from build123d import *

# Parameters (mm, degrees)
SKETCH1_W           = 63
SKETCH1_H           = 65
BOSS_EXTRUDE1_DEPTH = 35
SKETCH4_W           = 13.85
SKETCH4_H           = 28
CUT_EXTRUDE1_DEPTH  = 81.26362829
SKETCH6_R           = 2.05
CUT_EXTRUDE2_DEPTH  = 35
SKETCH7_W           = 35.3
SKETCH7_H           = 20
CUT_EXTRUDE3_DEPTH  = 58.214508823
SKETCH5_W           = 43.787246082
SKETCH5_H           = 26.488580963
CUT_EXTRUDE4_DEPTH  = 81.26362829
FILLET1_R           = 3
FILLET2_R           = 5


with BuildPart() as part:
    # Sketch1 → Boss-Extrude1 (new body)
    with BuildSketch(Plane.XY):
        Rectangle(SKETCH1_W, SKETCH1_H)
    extrude(amount=BOSS_EXTRUDE1_DEPTH)

    # Cut-Loft1: read off the stored shape, not the designer's step
    # Cut-Loft1: loft between two sections, ruled curve by curve
    cut_loft1_from = [
        Edge.make_bspline([(-16.5, -32.5, -15.95), (-16.5, -32.5, -14.245344374), (-16.5, -32.5, -10.830534175), (-16.5, -32.5, -5.7), (-16.5, -32.5, -0.569465825), (-16.5, -32.5, 2.845344374), (-16.5, -32.5, 5.208176172), (-16.24079277, -32.5, 6.487165764), (-15.189486136, -32.5, 8.102764154), (-13.584460954, -32.5, 9.238586175), (-12.225257815, -32.5, 9.55), (-9.654092683, -32.5, 9.55), (-5.862169747, -32.5, 9.55), (0, -32.5, 9.55), (5.862169747, -32.5, 9.55), (9.654092683, -32.5, 9.55), (12.225257815, -32.5, 9.55), (13.584460954, -32.5, 9.238586175), (15.189486136, -32.5, 8.102764154), (16.24079277, -32.5, 6.487165764), (16.5, -32.5, 5.208176172), (16.5, -32.5, 4.55)], [0, 0, 0, 0, 0.090746911, 0.181493823, 0.272240734, 0.362987645, 0.362987645, 0.398025487, 0.43306333, 0.468101172, 0.503139015, 0.503139015, 0.592316419, 0.681493823, 0.770671227, 0.859848631, 0.859848631, 0.894886473, 0.929924315, 0.964962158, 1, 1, 1, 1], 3),
        Edge.make_line((16.5, -32.5, 0), (16.5, -32.5, 4.55)),
        Edge.make_line((16.5, -32.5, 0), (-16.5, -32.5, -15.95)),
    ]
    cut_loft1_to = [
        Edge.make_bspline([(-13.65, 32.5, -15.8), (-13.65, 32.5, -14.113380525), (-13.65, 32.5, -10.745084998), (-13.65, 32.5, -5.7), (-13.65, 32.5, -0.654915002), (-13.65, 32.5, 2.713380525), (-13.65, 32.5, 5.051212323), (-13.38927185, 32.5, 6.394463384), (-12.20097724, 32.5, 8.116532102), (-10.480556624, 32.5, 9.187425671), (-9.241272853, 32.5, 9.4), (-7.145107721, 32.5, 9.4), (-4.236047985, 32.5, 9.4), (0, 32.5, 9.4), (4.236047985, 32.5, 9.4), (7.145107721, 32.5, 9.4), (9.241272853, 32.5, 9.4), (10.480556624, 32.5, 9.187425671), (12.20097724, 32.5, 8.116532102), (13.38927185, 32.5, 6.394463384), (13.65, 32.5, 5.051212323), (13.65, 32.5, 4.4)], [0, 0, 0, 0, 0.090746911, 0.181493823, 0.272240734, 0.362987645, 0.362987645, 0.398025487, 0.43306333, 0.468101172, 0.503139015, 0.503139015, 0.592316419, 0.681493823, 0.770671227, 0.859848631, 0.859848631, 0.894886473, 0.929924315, 0.964962158, 1, 1, 1, 1], 3),
        Edge.make_line((13.65, 32.5, 0), (13.65, 32.5, 4.4)),
        Edge.make_line((13.65, 32.5, 0), (-13.65, 32.5, -15.8)),
    ]
    cut_loft1 = Solid(Shell([*[Face.make_surface_from_curves(cut_loft1_from[k], cut_loft1_to[k]) for k in range(3)], Face(Wire(cut_loft1_from)), Face(Wire(cut_loft1_to))]))
    add(cut_loft1, mode=Mode.SUBTRACT)

    # Sketch4 → Cut-Extrude1 (cut, through all)
    with BuildSketch(Plane(origin=(0, 32.5, 0), x_dir=(1, 0, 0), z_dir=(0, 1, 0))):
        with Locations((24.575, -21)):
            Rectangle(SKETCH4_W, SKETCH4_H)
        with Locations((-24.575, -21)):
            Rectangle(SKETCH4_W, SKETCH4_H)
    extrude(amount=-CUT_EXTRUDE1_DEPTH, mode=Mode.SUBTRACT)

    # Sketch6 → Cut-Extrude2 (cut)
    with BuildSketch(Plane(origin=(0, 0, 0), x_dir=(-1, 0, 0), z_dir=(0, 0, -1))):
        with Locations((-26.5, -18.5)):
            Circle(SKETCH6_R)
        with Locations((-26.5, 1.5)):
            Circle(SKETCH6_R)
        with Locations((-26.5, 21.5)):
            Circle(SKETCH6_R)
        with Locations((26.5, -18.5)):
            Circle(SKETCH6_R)
        with Locations((26.5, 1.5)):
            Circle(SKETCH6_R)
        with Locations((26.5, 21.5)):
            Circle(SKETCH6_R)
    extrude(amount=-CUT_EXTRUDE2_DEPTH, mode=Mode.SUBTRACT)

    # Sketch7 → Cut-Extrude3 (cut, through all)
    with BuildSketch(Plane.XY.offset(35)):
        with Locations((0, -22.5)):
            Rectangle(SKETCH7_W, SKETCH7_H)
    extrude(amount=-CUT_EXTRUDE3_DEPTH, mode=Mode.SUBTRACT)

    # Sketch5 → Cut-Extrude4 (cut, through all)
    with BuildSketch(Plane(origin=(0, 32.5, 0), x_dir=(1, 0, 0), z_dir=(0, 1, 0))):
        with Locations((-0.216233314, -27.644290482)):
            Rectangle(SKETCH5_W, SKETCH5_H)
    extrude(amount=-CUT_EXTRUDE4_DEPTH, mode=Mode.SUBTRACT)

    # Fillet1
    fillet1_edges = [part.edges().sort_by_distance(p)[0] for p in [
        (17.65, 10, 7),
        (-17.65, 10, 7),
    ]]
    fillet(fillet1_edges, radius=FILLET1_R)

    # Fillet2
    fillet2_edges = [part.edges().sort_by_distance(p)[0] for p in [
        (-17.65, 10, 14.4),
        (17.65, 10, 14.4),
    ]]
    fillet(fillet2_edges, radius=FILLET2_R)


solid = part.part
Work out the finished part from the listing and answer in its coordinate system (mm). A direction names the side the tool comes from. Give positions to 0.01 mm unless a question says otherwise; leave off trailing zeros. Order: outer loops, then holes, each group sorted by start corner. A loop starts at its lowest first (then second) coordinate and runs counter-clockwise, first axis right, second up. Notation, with made-up numbers: (-36, 7.5) -> (4, 7.5) arc R33 ccw to (4, 46.5) -> close; hole circle Ø2 at (10, 2.25). An arc over 180 degrees is marked (long way). One line per item, written item: value.
Item 1: Determine the mould class of faces 3 (the cylindrical face through (28, -17.1, 3.5)), 4 (the flat face through (0, 10, 14.4)), 5 (the flat face through (-25, -32.5, 3)), 6 (the cylindrical face through (-24.45, 1.59, 3.45)) for opening direction Y: released by +Y, released by -Y, zero draft, split by the parting line, or undercut.
Answer sheet:
face 3: undercut
face 4: zero draft
face 5: released by -Y
face 6: undercut
Item 2: Straight lines are drawn through the part: probe 1 along Y at (x, z) = (-26.5, 3); probe 2 along X at (y, z) = (-25, 4); probe 3 along Y at (x, z) = (16, 2.25). For each, find the intervals that lie inside material, in ascending order.
Answer sheet:
probe 1: -32.5 to -20.55, -16.45 to -0.55, 3.55 to 19.45, 23.55 to 32.5
probe 2: -31.5 to -17.65, 17.65 to 31.5
probe 3: -12.5 to 32.5
Item 3: Find section A-A, the plane y = -18.5. Give the vertices of the cut face in (x, z), plus the area to 4 significant figures.
Answer sheet:
outline: (-31.5, 0) -> (-28.55, 0) -> (-28.55, 7) -> (-31.5, 7) -> close; (-24.45, 0) -> (-17.65, 0) -> (-17.65, 7) -> (-24.45, 7) -> close; (17.65, 0) -> (24.45, 0) -> (24.45, 7) -> (17.65, 7) -> close; (28.55, 0) -> (31.5, 0) -> (31.5, 7) -> (28.55, 7) -> close
area: 136.5 mm²
Item 4: A tool of negligible diameter and unlimited length cuts with its end or side. For faces 1 (the flat face through (-23, 0, 0)), 2 (the flat face through (-17.65, -23, 4)), from which of +Z, -Z, +X, -X, +Y, -Y can it reach the whole face along a straight path? Write none if from no direction.
Answer sheet:
face 1: -Z, +X, -X, +Y, -Y
face 2: +Z, -Z, -Y
Item 5: Find section B-B, the plane x = 26.5. Give the vertices of the cut face in (y, z), plus the area to 3 significant figures.
Answer sheet:
outline: (-32.5, 0) -> (-20.55, 0) -> (-20.55, 7) -> (-32.5, 7) -> close; (-16.45, 0) -> (-0.55, 0) -> (-0.55, 7) -> (-16.45, 7) -> close; (3.55, 0) -> (19.45, 0) -> (19.45, 7) -> (3.55, 7) -> close; (23.55, 0) -> (32.5, 0) -> (32.5, 7) -> (23.55, 7) -> close
area: 369 mm²
Item 6: Flat-ended cylindrical pins translate along their axes: P1, Ø4.5, axis at x = 3.5, z = 6.5, coming from the -Y side; P2, Ø7, axis at x = -24.5, y = 9.5, coming from the +Z side; P3, Ø6.5, axis at x = -26.5, y = -18.5, coming from the -Z side; P4, Ø2, axis at y = 17.5, z = 12, coming from the -X side. Find the tip coordinate at first contact, or state that the pin passes through.
Answer sheet:
P1: through
P2: z = 7
P3: z = 0
P4: x = -17.41
Item 7: Find section C-C, the plane y = 1.5. State how many separate pieces and enclosed holes the cut face has, plus the area to 3 significant figures.
Answer sheet:
separate pieces: 3
enclosed holes: 0
area: 365 mm²
